Check sheet for the modelled part. Datum: model origin and axes. Units: mm. Round coordinates to 2 decimals unless told otherwise and drop trailing zeros. Loops run counter-clockwise (first coordinate to the right, second up) from the corner with the lowest first, then second, coordinate; pieces in that order, holes last. Notation, with made-up numbers: M 28.25,81 L 72.25,81 A19 cw 72.25,85 Z; hole C -36.5,73.5 d6. An arc over 180 degrees is marked long. One line per question, with ' | ' between items. Start each with the question number.
(1) Section check A-A (x = 3). Record the boundary of the cut face in (y, z).
(2) Section check C-C (x = 10). Record the boundary of the cut face in (y, z).
(3) Thickness scan on probe 1 along Z at (x, y) = (24, -71.5); probe 2 along X at (y, z) = (-73.5, 32); probe 3 along Z at (x, y) = (0, -74.25). Record the ranges inside material, lowest first. Write a range as [from, to].
(4) Go/stop test with a flat-tipped pin: P1, Ø10, axis at x = 18, z = 5.5, coming from the -Y side. Record where the tip stops, or that it passes through.
(5) Section check B-B (z = 34). Record the boundary of the cut face in (x, y).
(6) Section check D-D (z = 26.5). Record the boundary of the cut face in (x, y).
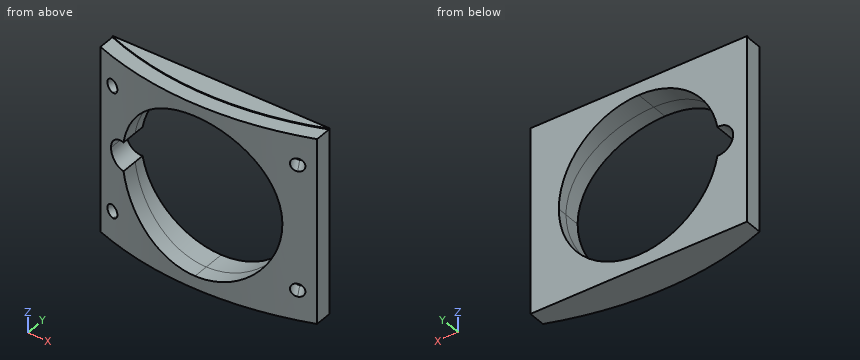
```python
from build123d import *

# Parameters (mm, degrees)
F0_R           = 78.74
F0_R_2         = 74.93
F1_DEPTH       = 38.1
F2_R           = 1.5875
F3_DEPTH       = 177.8
F7_DEPTH       = 25.4
F8_W           = 170.1503526419
F8_H           = 177.0643368363
F9_DEPTH       = 76.2
F12_END_RADIUS = 74.93
F12_REACH      = 113.8647376176
F13_DEPTH      = 69.85
F15_DEPTH      = 8.8910001


with BuildPart() as f1:
    # F0 (on Top) → F1 (new body, symmetric)
    with BuildSketch(Plane.XY):
        Circle(F0_R)
        Circle(F0_R_2, mode=Mode.SUBTRACT)
    extrude(amount=F1_DEPTH, both=True)

    # F2 (on Front) → F3 (intersect)
    with BuildSketch(Plane.XZ):
        with BuildLine():
            ThreePointArc((-19.685, 15.4305), (-13.9193969877, 29.3498969877), (0, 35.1155))
            Line((0, 35.1155), (0, 38.2905))
            Line((0, 38.2905), (-26.6664084047, 38.2905))
            Line((-26.6664084047, 38.2905), (-26.6664084047, 15.4305))
            Line((-26.6664084047, 15.4305), (-19.685, 15.4305))
        make_face()
        with Locations((-23.8125, 30.861)):
            Circle(F2_R, mode=Mode.SUBTRACT)
        with BuildLine():
            Line((0, -7.4295), (0, -4.2545))
            ThreePointArc((0, -4.2545), (-13.9193969877, 1.5111030123), (-19.685, 15.4305))
            Line((-19.685, 15.4305), (-26.6664084047, 15.4305))
            Line((-26.6664084047, 15.4305), (-26.6664084047, -7.4295))
            Line((-26.6664084047, -7.4295), (0, -7.4295))
        make_face()
        with Locations((-23.8125, 0)):
            Circle(F2_R, mode=Mode.SUBTRACT)
        with BuildLine():
            Line((26.6664084047, 15.4305), (19.685, 15.4305))
            ThreePointArc((19.685, 15.4305), (13.9193969877, 1.5111030123), (0, -4.2545))
            Line((0, -4.2545), (0, -7.4295))
            Line((0, -7.4295), (26.6664084047, -7.4295))
            Line((26.6664084047, -7.4295), (26.6664084047, 15.4305))
        make_face()
        with Locations((23.8125, 0)):
            Circle(F2_R, mode=Mode.SUBTRACT)
        with BuildLine():
            ThreePointArc((0, 35.1155), (13.9193969877, 29.3498969877), (19.685, 15.4305))
            Line((19.685, 15.4305), (26.6664084047, 15.4305))
            Line((26.6664084047, 15.4305), (26.6664084047, 38.2905))
            Line((26.6664084047, 38.2905), (0, 38.2905))
            Line((0, 38.2905), (0, 35.1155))
        make_face()
        with Locations((23.8125, 30.861)):
            Circle(F2_R, mode=Mode.SUBTRACT)
        with Locations((-23.8125, 30.861)):
            Circle(F2_R)
        with Locations((23.8125, 30.861)):
            Circle(F2_R)
        with Locations((-23.8125, 0)):
            Circle(F2_R)
        with Locations((23.8125, 0)):
            Circle(F2_R)
    extrude(amount=F3_DEPTH, mode=Mode.INTERSECT)

    # F6 (on face) → F7 (cut)
    with BuildSketch(Plane(origin=(38.7472337077, -67.1121774345, 0), x_dir=(-0.8660254038, -0.5, 0), z_dir=(-0.5, 0.8660254038, 0))):
        with BuildLine():
            ThreePointArc((19.5060294768, 0), (19.041061492, 1.1225320151), (17.9185294768, 1.5875))
            Line((17.9185294768, 1.5875), (17.9185294768, -1.5875))
            ThreePointArc((17.9185294768, -1.5875), (19.041061492, -1.1225320151), (19.5060294768, 0))
        make_face()
        with BuildLine():
            Line((17.9185294768, -1.5875), (17.9185294768, 1.5875))
            ThreePointArc((17.9185294768, 1.5875), (16.3310294768, 0), (17.9185294768, -1.5875))
        make_face()
        with BuildLine():
            ThreePointArc((19.5060294768, 30.861), (19.041061492, 31.9835320151), (17.9185294768, 32.4485))
            Line((17.9185294768, 32.4485), (17.9185294768, 29.2735))
            ThreePointArc((17.9185294768, 29.2735), (19.041061492, 29.7384679849), (19.5060294768, 30.861))
        make_face()
        with BuildLine():
            Line((17.9185294768, 29.2735), (17.9185294768, 32.4485))
            ThreePointArc((17.9185294768, 32.4485), (16.3310294768, 30.861), (17.9185294768, 29.2735))
        make_face()
    extrude(amount=F7_DEPTH, mode=Mode.SUBTRACT)

    # F8 (on Right) → F9 (cut)
    with BuildSketch(Plane.YZ):
        with Locations((-62.6385295764, 18.013317138)):
            Rectangle(F8_W, F8_H)
    extrude(amount=-F9_DEPTH, mode=Mode.SUBTRACT)

    # F10: F1 across plane


with BuildPart() as f1_1:
    add(f1.part)
    add(f1.part.mirror(Plane.YZ))

    f12_end = (Plane(origin=(0, 0, 15.33525), x_dir=(-1, 0, 0), z_dir=(0, 0, -1)) * Cylinder(F12_END_RADIUS, 369.0558714917, mode=Mode.PRIVATE)).faces().sort_by_distance((0, -74.93, -6.7265497667))[0]
    # F2 (on Front) → F12 (join, up to the whole of a round face its end follows)
    with BuildSketch(Plane.XZ):
        with BuildLine():
            ThreePointArc((0, 35.1155), (13.9193969877, 29.3498969877), (19.685, 15.4305))
            Line((19.685, 15.4305), (26.6664084047, 15.4305))
            Line((26.6664084047, 15.4305), (26.6664084047, 38.2905))
            Line((26.6664084047, 38.2905), (0, 38.2905))
            Line((0, 38.2905), (0, 35.1155))
        make_face()
        with Locations((23.8125, 30.861)):
            Circle(F2_R, mode=Mode.SUBTRACT)
        with BuildLine():
            ThreePointArc((-19.685, 15.4305), (-13.9193969877, 29.3498969877), (0, 35.1155))
            Line((0, 35.1155), (0, 38.2905))
            Line((0, 38.2905), (-26.6664084047, 38.2905))
            Line((-26.6664084047, 38.2905), (-26.6664084047, 15.4305))
            Line((-26.6664084047, 15.4305), (-19.685, 15.4305))
        make_face()
        with Locations((-23.8125, 30.861)):
            Circle(F2_R, mode=Mode.SUBTRACT)
        with BuildLine():
            Line((0, -7.4295), (0, -4.2545))
            ThreePointArc((0, -4.2545), (-13.9193969877, 1.5111030123), (-19.685, 15.4305))
            Line((-19.685, 15.4305), (-26.6664084047, 15.4305))
            Line((-26.6664084047, 15.4305), (-26.6664084047, -7.4295))
            Line((-26.6664084047, -7.4295), (0, -7.4295))
        make_face()
        with Locations((-23.8125, 0)):
            Circle(F2_R, mode=Mode.SUBTRACT)
        with BuildLine():
            Line((26.6664084047, 15.4305), (19.685, 15.4305))
            ThreePointArc((19.685, 15.4305), (13.9193969877, 1.5111030123), (0, -4.2545))
            Line((0, -4.2545), (0, -7.4295))
            Line((0, -7.4295), (26.6664084047, -7.4295))
            Line((26.6664084047, -7.4295), (26.6664084047, 15.4305))
        make_face()
        with Locations((23.8125, 0)):
            Circle(F2_R, mode=Mode.SUBTRACT)
        with Locations((-23.8125, 0)):
            Circle(F2_R)
        with Locations((-23.8125, 30.861)):
            Circle(F2_R)
        with Locations((23.8125, 30.861)):
            Circle(F2_R)
        with Locations((23.8125, 0)):
            Circle(F2_R)
    f12_long = extrude(amount=F12_REACH, mode=Mode.PRIVATE)
    add(split(f12_long, bisect_by=f12_end, keep=Keep.BOTTOM, mode=Mode.PRIVATE))

    # F2 (on Front) → F13 (cut)
    with BuildSketch(Plane.XZ):
        with BuildLine():
            Line((26.6664084047, 15.4305), (19.685, 15.4305))
            ThreePointArc((19.685, 15.4305), (13.9193969877, 1.5111030123), (0, -4.2545))
            Line((0, -4.2545), (0, -7.4295))
            Line((0, -7.4295), (26.6664084047, -7.4295))
            Line((26.6664084047, -7.4295), (26.6664084047, 15.4305))
        make_face()
        with Locations((23.8125, 0)):
            Circle(F2_R, mode=Mode.SUBTRACT)
        with BuildLine():
            ThreePointArc((-19.685, 15.4305), (-13.9193969877, 29.3498969877), (0, 35.1155))
            Line((0, 35.1155), (0, 38.2905))
            Line((0, 38.2905), (-26.6664084047, 38.2905))
            Line((-26.6664084047, 38.2905), (-26.6664084047, 15.4305))
            Line((-26.6664084047, 15.4305), (-19.685, 15.4305))
        make_face()
        with Locations((-23.8125, 30.861)):
            Circle(F2_R, mode=Mode.SUBTRACT)
        with BuildLine():
            Line((0, -7.4295), (0, -4.2545))
            ThreePointArc((0, -4.2545), (-13.9193969877, 1.5111030123), (-19.685, 15.4305))
            Line((-19.685, 15.4305), (-26.6664084047, 15.4305))
            Line((-26.6664084047, 15.4305), (-26.6664084047, -7.4295))
            Line((-26.6664084047, -7.4295), (0, -7.4295))
        make_face()
        with Locations((-23.8125, 0)):
            Circle(F2_R, mode=Mode.SUBTRACT)
        with BuildLine():
            ThreePointArc((0, 35.1155), (13.9193969877, 29.3498969877), (19.685, 15.4305))
            Line((19.685, 15.4305), (26.6664084047, 15.4305))
            Line((26.6664084047, 15.4305), (26.6664084047, 38.2905))
            Line((26.6664084047, 38.2905), (0, 38.2905))
            Line((0, 38.2905), (0, 35.1155))
        make_face()
        with Locations((23.8125, 30.861)):
            Circle(F2_R, mode=Mode.SUBTRACT)
        with Locations((-23.8125, 0)):
            Circle(F2_R)
        with Locations((23.8125, 0)):
            Circle(F2_R)
        with Locations((23.8125, 30.861)):
            Circle(F2_R)
        with Locations((-23.8125, 30.861)):
            Circle(F2_R)
    extrude(amount=F13_DEPTH, mode=Mode.SUBTRACT)

    # F14 (on face) → F15 (cut, through all)
    with BuildSketch(Plane(origin=(0, -69.85, 0), x_dir=(-1, 0, 0), z_dir=(0, 1, 0))):
        with BuildLine():
            ThreePointArc((19.3638129032, 18.971965071), (19.6045387857, 17.2085), (19.685, 15.4305))
            ThreePointArc((19.685, 15.4305), (19.6045387857, 13.6525), (19.3638129032, 11.889034929))
            ThreePointArc((19.3638129032, 11.889034929), (22.0832279587, 12.8049260326), (23.241, 15.4305))
            ThreePointArc((23.241, 15.4305), (22.0832279587, 18.0560739674), (19.3638129032, 18.971965071))
        make_face()
        with BuildLine():
            ThreePointArc((19.3638129032, 11.889034929), (19.6045387857, 13.6525), (19.685, 15.4305))
            Line((19.685, 15.4305), (16.129, 15.4305))
            ThreePointArc((16.129, 15.4305), (17.0594260326, 13.0322720413), (19.3638129032, 11.889034929))
        make_face()
    extrude(amount=-F15_DEPTH, mode=Mode.SUBTRACT)


solid = f1_1.part
```
The answers:
1) outline: M -78.68,-7.43 L -69.85,-7.43 L -69.85,-4.02 L -78.68,-4.02 Z; M -78.68,34.89 L -69.85,34.89 L -69.85,38.29 L -74.87,38.29 L -74.87,38.1 L -78.68,38.1 Z
2) outline: M -78.1,-7.43 L -69.85,-7.43 L -69.85,-1.53 L -78.1,-1.53 Z; M -78.1,32.39 L -69.85,32.39 L -69.85,38.29 L -74.26,38.29 L -74.26,38.1 L -78.1,38.1 Z
3) probe 1: [-7.43, 38.1] | probe 2: [-26.67, -23.02], [-20.47, -10.63], [10.63, 20.47], [23.02, 26.67] | probe 3: [-7.43, -4.25], [35.12, 38.29]
4) P1: y = -77.41
5) outline: M -26.67,-74.09 A78.74 ccw -6.53,-78.47 L -6.53,-69.85 L -26.67,-69.85 Z; M 6.53,-78.47 A78.74 ccw 26.67,-74.09 L 26.67,-69.85 L 6.53,-69.85 Z
6) outline: M -26.67,-74.09 A78.74 ccw -16.28,-77.04 L -16.28,-69.85 L -26.67,-69.85 Z; M 16.28,-77.04 A78.74 ccw 26.67,-74.09 L 26.67,-69.85 L 16.28,-69.85 Z
